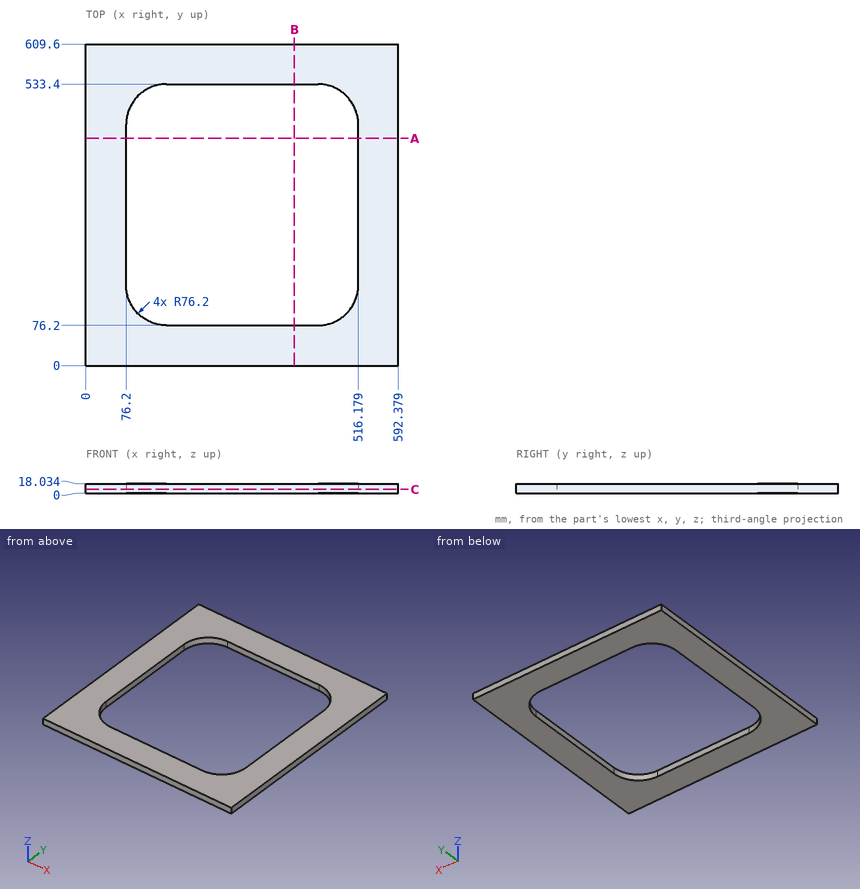
Design review of the part shown in the three views and the two pictorial views. Dimensions are in mm from the part's minimum x, y and z. Give positions to 0.01 mm unless a question says otherwise; leave off trailing zeros. Loops run counter-clockwise (first coordinate to the right, second up) from the corner with the lowest first, then second, coordinate; pieces in that order, holes last. Notation, with made-up numbers: M 79.5,20.5 L 116.5,20.5 A13 cw 116.5,43.5 Z; hole C 81,5 d1. An arc over 180 degrees is marked long. Put each result on its own line as item: value. Start each with the question number.
(1) Add section C-C, the plane z = 6.75. Write out the cut boundary in (x, y), then the cut area to 3 significant figures.
(2) Add section B-B, the plane x = 395. Write out the cut boundary in (y, z).
(3) Wall thickness on L1, parallel to X at y = 314, z = 1.5; L2, parallel to Y at x = 415.5, z = 9.25; L3, parallel to X at y = 521.5, z = 14: over which ranges is each line inside the solid? List them lowest first.
(4) Add section A-A, the plane y = 430.5. Write out the cut boundary in (x, z).
Result:
1. outline: M 0,0 L 592.38,0 L 592.38,609.6 L 0,609.6 Z; hole M 76.2,152.4 A76.2 ccw 152.4,76.2 L 439.98,76.2 A76.2 ccw 516.18,152.4 L 516.18,457.2 A76.2 ccw 439.98,533.4 L 152.4,533.4 A76.2 ccw 76.2,457.2 Z
1. area: 165,000 mm^2
2. outline: M 0,0 L 76.2,0 L 76.2,18.03 L 0,18.03 Z; M 533.4,0 L 609.6,0 L 609.6,18.03 L 533.4,18.03 Z
3. L1: x = 0 to 76.2, 516.18 to 592.38
3. L2: y = 0 to 76.2, 533.4 to 609.6
3. L3: x = 0 to 111.51, 480.87 to 592.38
4. outline: M 0,0 L 76.2,0 L 76.2,18.03 L 0,18.03 Z; M 516.18,0 L 592.38,0 L 592.38,18.03 L 516.18,18.03 Z
